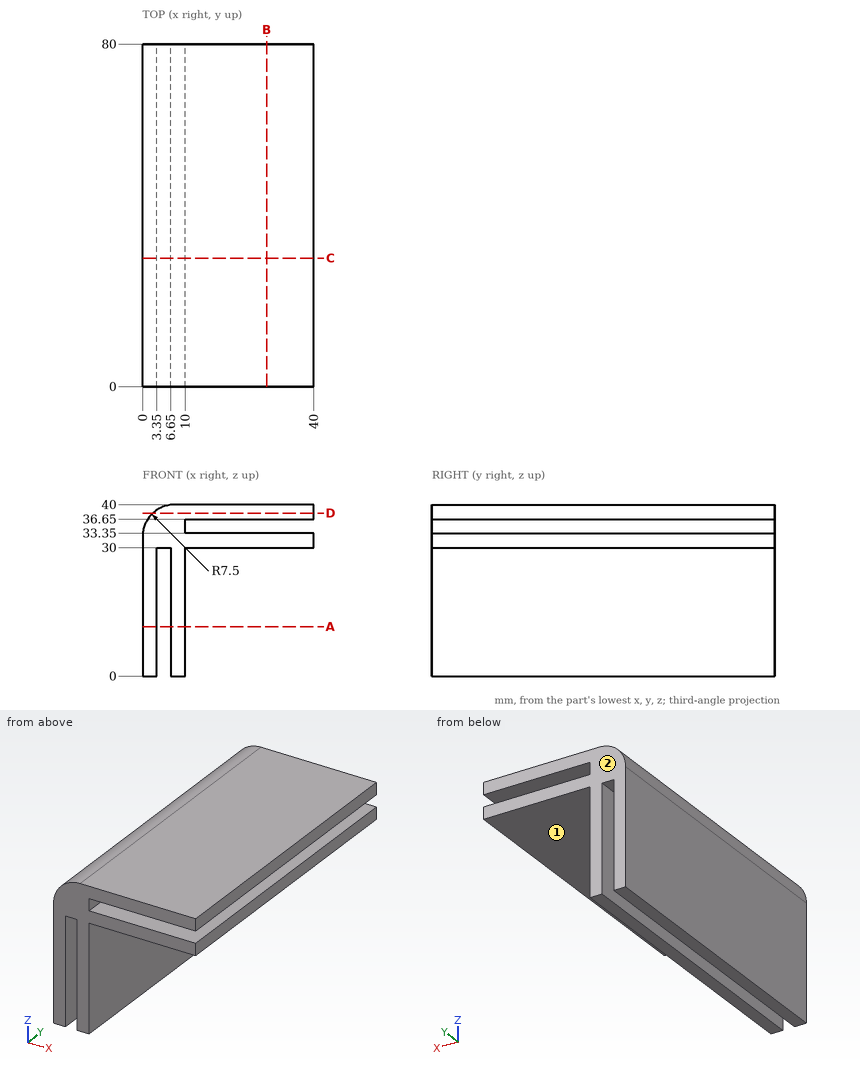
Input: dimensioned drawing with shaded views. Units: mm. Origin: part minimum x, y, z. A direction names the side the tool comes from. Give positions to 0.01 mm unless a question says otherwise; leave off trailing zeros. Loops run counter-clockwise (first coordinate to the right, second up) from the corner with the lowest first, then second, coordinate; pieces in that order, holes last. Notation, with made-up numbers: (34, -20.5) -> (61, -20.5) arc R33 cw to (61, 8.5) -> close; hole circle Ø5 at (6, 42). An arc over 180 degrees is marked (long way). Return JSON: item names as keys, results as strings.
Item 1: Section B-B, the plane x = 29. Output: boundary loops of the cut face in (y, z).
Filled in:
{"outline": "(0, 30) -> (80, 30) -> (80, 33.35) -> (0, 33.35) -> close; (0, 36.65) -> (80, 36.65) -> (80, 40) -> (0, 40) -> close"}
Item 2: Section C-C, the plane y = 30. Output: boundary loops of the cut face in (x, z).
Filled in:
{"outline": "(0, 0) -> (3.35, 0) -> (3.35, 30) -> (6.65, 30) -> (6.65, 0) -> (10, 0) -> (10, 30) -> (40, 30) -> (40, 33.35) -> (10, 33.35) -> (10, 36.65) -> (40, 36.65) -> (40, 40) -> (7.5, 40) arc R7.5 ccw to (0, 32.5) -> close"}
Item 3: Pin query (flat end, axial travel): P1, Ø1.5, axis at x = 33.5, z = 27.5, coming from the -Y side; P2, Ø1, axis at x = 5.5, y = 31.5, coming from the -Z side; P3, Ø1.5, axis at y = 28.5, z = 28.5, coming from the +X side. Return the tip coordinate at first contact, or that it passes through.
Filled in:
{"P1": "through", "P2": "z = 30", "P3": "x = 10"}
Item 4: Access query for the marked faces 1 and 2. Directions: +Z, -Z, +X, -X, +Y, -Y. A direction counts if a zero-diameter tool reaches every point of the face in a straight line with its end or side. Return the directions, or none.
Filled in:
{"face 1": "-Z, +X, +Y, -Y", "face 2": "+Z, -Z, +X, -X, +Y"}
Item 5: Section A-A, the plane z = 11.5. Output: boundary loops of the cut face in (x, y).
Filled in:
{"outline": "(0, 0) -> (3.35, 0) -> (3.35, 80) -> (0, 80) -> close; (6.65, 0) -> (10, 0) -> (10, 80) -> (6.65, 80) -> close"}
Item 6: Line query: line 1 (Z direction, x = 15.5, y = 10.5); line 2 (X direction, y = 38.5, z = 13); line 3 (X direction, y = 75, z = 37.5). Output: solid intervals per line, ascending.
Filled in:
{"line 1": "30 to 33.35, 36.65 to 40", "line 2": "0 to 3.35, 6.65 to 10", "line 3": "1.91 to 40"}
Item 7: Section D-D, the plane z = 38. Output: boundary loops of the cut face in (x, y).
Filled in:
{"outline": "(2.4, 0) -> (40, 0) -> (40, 80) -> (2.4, 80) -> close"}
